```python
from build123d import *

# Parameters (mm, degrees)
BOSS_EXTRUDE2_DEPTH = 10
BOSS_EXTRUDE3_DEPTH = 310
SKETCH7_W           = 290
SKETCH7_H           = 40
CUT_EXTRUDE1_DEPTH  = 589


with BuildPart() as part:
    # Sketch2 → Boss-Extrude2 (new body)
    with BuildSketch(Plane(origin=(0, 0, 0), x_dir=(1, 0, 0), z_dir=(0, 1, 0))):
        with BuildLine():
            Line((200, 155), (245.398448916, 109.601551084))
            ThreePointArc((245.398448916, 109.601551084), (510, 0), (245.398448916, -109.601551084))
            Line((245.398448916, -109.601551084), (200, -155))
            Line((200, -155), (-200, -155))
            Line((-200, -155), (-200, 155))
            Line((-200, 155), (200, 155))
        make_face()
    extrude(amount=BOSS_EXTRUDE2_DEPTH)

    # Sketch6 → Boss-Extrude3 (add)
    with BuildSketch(Plane.XY.offset(155)):
        with BuildLine():
            Line((-35, 10), (-55, 10))
            Line((-55, 10), (-55, -30))
            ThreePointArc((-55, -30), (-45, -40), (-35, -30))
            Line((-35, -30), (-35, 10))
        make_face()
        with BuildLine():
            Line((365, 10), (345, 10))
            Line((345, 10), (345, -30))
            ThreePointArc((345, -30), (355, -40), (365, -30))
            Line((365, -30), (365, 10))
        make_face()
    extrude(amount=-BOSS_EXTRUDE3_DEPTH)

    # Sketch7 → Cut-Extrude1 (cut)
    with BuildSketch(Plane.ZY.offset(55)):
        with Locations((0, -20)):
            Rectangle(SKETCH7_W, SKETCH7_H)
    extrude(amount=-CUT_EXTRUDE1_DEPTH, mode=Mode.SUBTRACT)


solid = part.part
```
Source: CAD feature listing. Evaluate the final solid. Frame: model axes, mm. A direction names the side the tool comes from. Round coordinates to 2 decimals unless told otherwise and drop trailing zeros. Loops run counter-clockwise (first coordinate to the right, second up) from the corner with the lowest first, then second, coordinate; pieces in that order, holes last.
(1) Section query D-D (z = 64). Output: boundary loops of the cut face in (x, y).
From the geometry:
outline: (-200, 0) - (496.17, 0) - (496.17, 10) - (-200, 10) - close
(2) Access query for faces 5 (the flat face through (223, 5, 132)), 6 (the flat face through (222, 5, -133)), 7 (the flat face through (355, -20, -145)), 8 (the flat face through (355, -15, -155)). Directions: +Z, -Z, +X, -X, +Y, -Y. A direction counts if a zero-diameter tool reaches every point of the face in a straight line with its end or side. Return the directions, or none.
From the geometry:
face 5: +Z, +Y, -Y
face 6: -Z, +Y, -Y
face 7: +X, -X, -Y
face 8: -Z, +X, -X, +Y, -Y
(3) Contact query for flat-ended pins moving along their axis: pin 1 Ø3 at (y, z) = (-20, 150) entering from +X; pin 2 Ø6 at (y, z) = (-5.5, -17.5) entering from +X; pin 3 Ø3 at (y, z) = (-16.5, 150) entering from -X; pin 4 Ø8 at (y, z) = (-0.5, 79.5) entering from +X. Output: stop coordinate, or through.
From the geometry:
pin 1: stops at x = 365
pin 2: passes through
pin 3: stops at x = -55
pin 4: stops at x = 490.35
(4) Section query B-B (x = -45). Output: boundary loops of the cut face in (y, z).
From the geometry:
outline: (-40, -155) - (10, -155) - (10, 155) - (-40, 155) - (-40, 145) - (0, 145) - (0, -145) - (-40, -145) - close
(5) Section query A-A (y = -17). Output: boundary loops of the cut face in (x, z), and give its area (3 significant figures).
From the geometry:
outline: (-55, -155) - (-35, -155) - (-35, -145) - (-55, -145) - close; (-55, 145) - (-35, 145) - (-35, 155) - (-55, 155) - close; (345, -155) - (365, -155) - (365, -145) - (345, -145) - close; (345, 145) - (365, 145) - (365, 155) - (345, 155) - close
area: 800 mm2
(6) Section query C-C (z = 0). Output: boundary loops of the cut face in (x, y), and give its area (3 significant figures).
From the geometry:
outline: (-200, 0) - (510, 0) - (510, 10) - (-200, 10) - close
area: 7,100 mm2
(7) Material intervals for probe 1 along Y at (x, z) = (90, -89); probe 2 along X at (y, z) = (5, 5); probe 3 along Z at (x, y) = (477, 5), sorted ascending.
From the geometry:
probe 1: y = 0 to 10
probe 2: x = -200 to 509.92
probe 3: z = -95.61 to 95.61
(8) Pull-direction query (Z, two-part tool) for faces 1 (the flat face through (-45, -20, -145)), 2 (the cylindrical face through (509.966, 4.93, -3.268)), 3 (the flat face through (-45, -20, 145)), 4 (the flat face through (1, 3, 155)); classes: +Z half, -Z half, draft (parallel to the pull), parting line (faces both ways), or undercut.
From the geometry:
face 1: undercut
face 2: parting line
face 3: undercut
face 4: +Z half
